Read the model definition and answer for the solid it produces. Units are mm, in the model's axes. Face numbers are marked on the shaded views. Give positions to 0.01 mm unless a question says otherwise; leave off trailing zeros. Order: outer loops, then holes, each group sorted by start corner. A loop starts at its lowest first (then second) coordinate and runs counter-clockwise, first axis right, second up.
Item 1: Find the intervals of material crossed by line 1 along X through (y, z) = (-95, -49); line 2 along Y through (x, z) = (20, 28); line 3 along X through (y, z) = (-13.5, -41), in increasing order.
Item 2: A cutting plane is placed at B-B (x = -19.5). Write down the section's boundary in (y, z).
Item 3: A cutting plane is placed at A-A (z = -55.5). Write down the section's boundary in (x, y), plus the area to 3 significant figures.
Item 4: The mould has two halves that part along Z. Classify the marked faces 1, 2, 3 and 4: +Z half, -Z half, draft (parallel to the pull), parting line (faces both ways), or undercut.
Item 5: Given pin 1 Ø1 at (x, z) = (69, 2) entering from +Y; pin 2 Ø2 at (x, z) = (-7, 10) entering from +Y; pin 3 Ø1 at (x, z) = (69, 3.5) entering from -Y; pin 4 Ø0.6 at (x, z) = (69, -8) entering from -Y, each flat-ended and moving along its own axis, determine where each tip first touches the part or whether it passes through.
Item 6: A cutting plane is placed at C-C (y = -12.5). Write down the section's boundary in (x, z), plus the area to 3 significant figures.
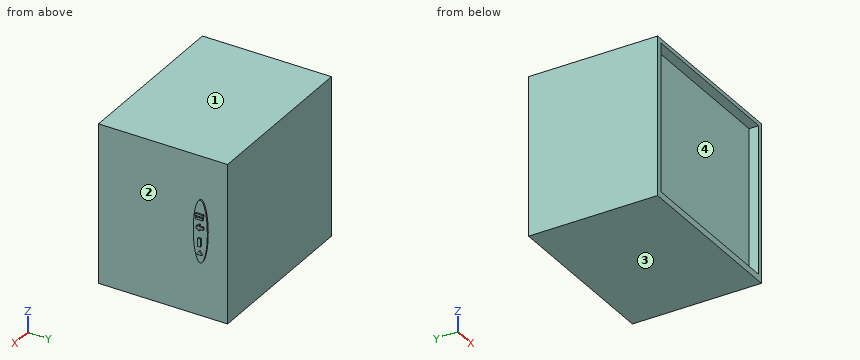
from build123d import *

# Parameters (mm, degrees)
F0_W      = 133.9241117239
F0_H      = 125.1133196056
F1_DEPTH  = 101.6
F2_W      = 126.0571889579
F2_H      = 116.7119294405
F3_DEPTH  = 7.62
F5_DEPTH  = 68.58
F6_W      = 6.050657481
F6_H      = 1.6052769497
F7_DEPTH  = 69.85
F8_W      = 5.8036912233
F8_H      = 1.6052750871
F9_DEPTH  = 69.85
F10_W     = 1.605277881
F10_H     = 1.975722611
F10_W_2   = 1.1730855331
F10_H_2   = 1.2348302407
F10_W_3   = 2.7783634141
F10_H_3   = 1.3583111577
F11_DEPTH = 69.85
F13_DEPTH = 69.85
F14_W     = 2.3461729288
F14_H     = 6.297617685
F15_DEPTH = 69.85


with BuildPart() as f1:
    # F0 (on Front) → F1 (new body)
    with BuildSketch(Plane.XZ):
        with Locations((0.4405379295, -3.9648581296)):
            Rectangle(F0_W, F0_H)
    extrude(amount=F1_DEPTH)

    # F2 (on face) → F3 (cut)
    with BuildSketch(Plane.XZ.offset(101.6)):
        with Locations((0.8558873087, -3.030333668)):
            Rectangle(F2_W, F2_H)
    extrude(amount=-F3_DEPTH, mode=Mode.SUBTRACT)

    # F4 (on Right) → F5 (join)
    with BuildSketch(Plane.YZ):
        with BuildLine():
            add(Edge.make_bspline(
                [(-20.7936801016, -24.5864875615), (-11.1313539485, -24.5864875615), (-15.9625170251, 12.2932437807), (-20.7936801016, 49.1729751229), (-25.6248431782, 12.2932437807), (-30.4560062548, -24.5864875615), (-20.7936801016, -24.5864875615)],
                knots=[0, 0, 0, 2.0943951024, 2.0943951024, 4.1887902048, 4.1887902048, 6.2831853072, 6.2831853072, 6.2831853072], degree=2, weights=[1, 0.5, 1, 0.5, 1, 0.5, 1]))
        make_face()
    extrude(amount=F5_DEPTH)

    # F6 (on Right) → F7 (join)
    with BuildSketch(Plane.YZ):
        with Locations((-21.0075564682, 13.3131914772)):
            Rectangle(F6_W, F6_H)
    extrude(amount=F7_DEPTH)

    # F8 (on Right) → F9 (join)
    with BuildSketch(Plane.YZ):
        with Locations((-21.0355212912, 10.5541222729)):
            Rectangle(F8_W, F8_H)
    extrude(amount=F9_DEPTH)

    # F10 (on Right) → F11 (join)
    with BuildSketch(Plane.YZ):
        with Locations((-22.6139808074, 3.4591723233)):
            Rectangle(F10_W, F10_H)
        with Locations((-21.2247991003, 3.4591723233)):
            Rectangle(F10_W_2, F10_H)
        with Locations((-21.2247991003, 1.8538958975)):
            Rectangle(F10_W_2, F10_H_2)
        with Locations((-19.2490746267, 3.4591723233)):
            Rectangle(F10_W_3, F10_H)
        with Locations((-21.2247991003, 5.1261892077)):
            Rectangle(F10_W_2, F10_H_3)
    extrude(amount=F11_DEPTH)

    # F12 (on Right) → F13 (join)
    with BuildSketch(Plane.YZ):
        Polygon((-20.9511611611, -14.6655198187), (-23.2355929911, -17.6291037351), (-18.666729331, -17.6291037351), align=None)
    extrude(amount=F13_DEPTH)

    # F14 (on Right) → F15 (join)
    with BuildSketch(Plane.YZ):
        with Locations((-21.0262555629, -8.1192564685)):
            Rectangle(F14_W, F14_H)
    extrude(amount=F15_DEPTH)


solid = f1.part
Response values:
1. line 1: x = -66.52 to -62.17, 63.88 to 67.4
1. line 2: y = -93.98 to 0
1. line 3: x = -66.52 to 67.4
2. outline: (-101.6, -66.52) - (0, -66.52) - (0, 58.59) - (-101.6, 58.59) - (-101.6, 55.33) - (-93.98, 55.33) - (-93.98, -61.39) - (-101.6, -61.39) - close
3. outline: (-66.52, -101.6) - (-62.17, -101.6) - (-62.17, -93.98) - (63.88, -93.98) - (63.88, -101.6) - (67.4, -101.6) - (67.4, 0) - (-66.52, 0) - close
3. area: 12,600 mm2
4. face 1: +Z half
4. face 2: draft
4. face 3: -Z half
4. face 4: undercut
5. pin 1: stops at y = -15.23
5. pin 2: stops at y = 0
5. pin 3: stops at y = -26.32
5. pin 4: stops at y = -22.2
6. outline: (-66.52, -66.52) - (67.4, -66.52) - (67.4, 58.59) - (-66.52, 58.59) - close
6. area: 16,800 mm2
